The drawing under review shows one solid part. Ordinate dimensions are in mm from its lowest x, y, z. A direction names the side the tool comes from. Give positions to 0.01 mm unless a question says otherwise; leave off trailing zeros. Write each loop counter-clockwise with the first axis right and the second up, starting at its lowest first coordinate (ties: lowest second). Pieces come first, ordered by that corner, then holes. Notation, with made-up numbers: (-3, 48.25) -> (27, 48.25) arc R11 cw to (27, 63.25) -> close; hole circle Ø11 at (-29, -7). An arc over 180 degrees is marked (long way). Answer as a JSON object with one key per item and string values.
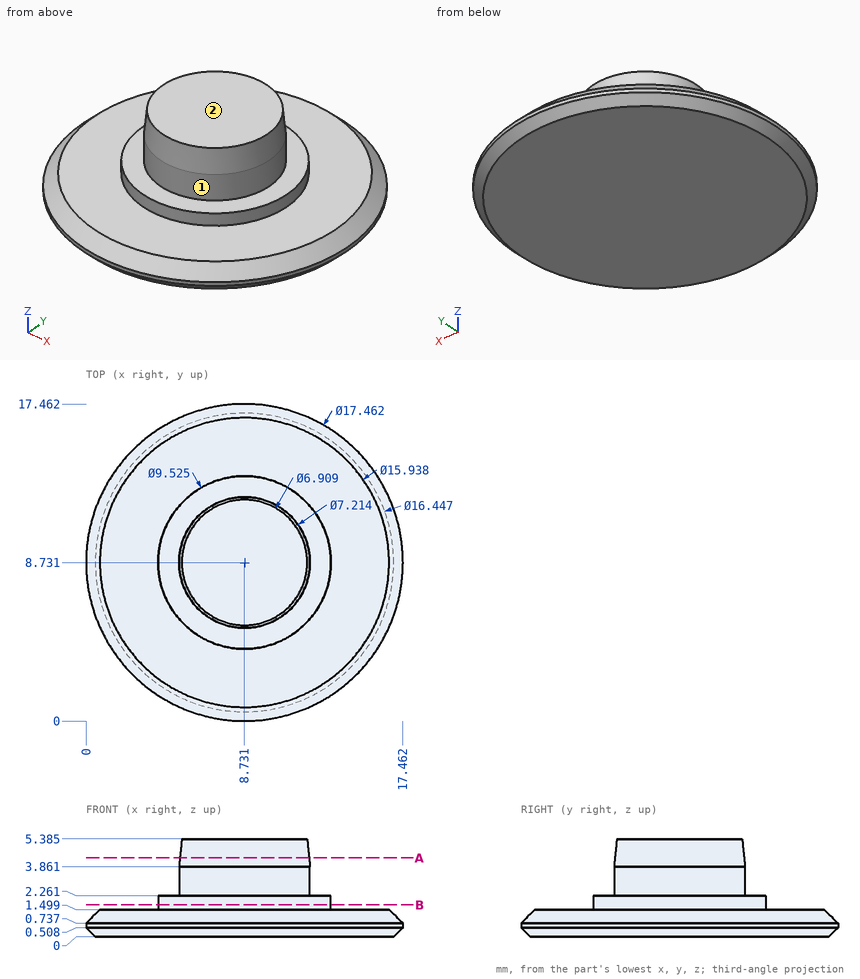
(1) For the marked faces 1 and 2, list the 3-axis set-ups (+Z, -Z, +X, -X, +Y, -Y) from which the entire face can be reached by the end or side of a thin tool; tool diameter is ignored.
Here are the results:
{"face 1": "+Z", "face 2": "+Z, +X, -X, +Y, -Y"}
(2) For line 1 along Z through (x, y) = (14, 3.5); line 2 along Z through (x, y) = (11, 5); line 3 along X through (y, z) = (6.75, 3.85) (1 decimal), list the stretches that pass through material, from the lowest coordinate up.
Here are the results:
{"line 1": "z = 0 to 1.5", "line 2": "z = 0 to 2.26", "line 3": "x = 5.7 to 11.7"}
(3) Clearance check with flat-ended pins moving along their axes: pin 1 (6 mm diameter, centred on x = 4, y = 15.5, fed in from +Z); pin 2 (1.5 mm diameter, centred on x = 5.5, z = 1, fed in from +Y); pin 3 (4 mm diameter, centred on x = 5.5, y = 2, fed in from -Z); pin 4 (1.5 mm diameter, centred on x = 10.5, z = 2, fed in from -Y). State where each tip first meets the part, or that it passes through.
Here are the results:
{"pin 1": "stops at z = 1.5", "pin 2": "stops at y = 17.09", "pin 3": "stops at z = 0", "pin 4": "stops at y = 0.69"}
(4) We need section A-A, the plane z = 4.35. State the section outline as (x, y) points (1 decimal).
Here are the results:
{"outline": "circle Ø7.1 at (8.7, 8.7)"}
(5) We need section B-B, the plane z = 1.75. State the section outline as (x, y) points (1 decimal).
Here are the results:
{"outline": "circle Ø9.5 at (8.7, 8.7)"}
